Could you check a few things on this model? Use its own coordinates, in mm. Face numbers are marked on the shaded views. A direction names the side the tool comes from. Coordinates: 2 decimals unless noted, no trailing zeros. Write each loop counter-clockwise with the first axis right and the second up, starting at its lowest first coordinate (ties: lowest second). Pieces come first, ordered by that corner, then holes. Notation, with made-up numbers: (-28.75, -4) - (10.25, -4) arc R33 ccw to (10.25, 24) - close; hole circle Ø7 at (-23.5, 62). An arc over 180 degrees is marked (long way). Answer as a JSON object with one key per item and string values. Group by question number.
1) If we section it at D-D (z = -4.75): Write out the boundary of the cut face in (x, y) (3 decimals).
2) Will these pins go through, and if not, where does the flat tip stop? pin 1 Ø4 at (x, z) = (5, -6.5) entering from +Y (3 decimals); pin 2 Ø1 at (x, y) = (15.5, 6.5) entering from +Z (3 decimals).
3) If we section it at C-C (y = 1.75): State how many separate pieces and enclosed holes the cut face has, plus the area to 3 significant figures.
4) We'd pull the mould along X, two halves only. Please class the marked faces 3, 4 and 5: released by +X, released by -X, zero draft, split by the parting line, or undercut.
5) If we section it at A-A (x = 12.7): Write out the boundary of the cut face in (y, z) (1 decimal), plus the area to 3 significant figures.
6) Please list where these lines run through material, in increasing order: line 1 along X through (y, z) = (1, -4.5); line 2 along Y through (x, z) = (12.7, -11.65) (1 decimal); line 3 along Z through (x, y) = (19.05, 0.8) (3 decimals).
7) If we section it at B-B (y = 5.08): Write out the boundary of the cut face in (x, z) (1 decimal).
8) On a 3-axis mill with a long thin cutter (end or side, diameter ignored), from which of +Z, -Z, +X, -X, +Y, -Y can I reach the whole of each face in a straight line? I mean the marked faces 1 and 2. Say none if no direction works.
```python
from build123d import *

# Parameters (mm, degrees)
SKETCH1_W           = 25.4
SKETCH1_H           = 12.7
BOSS_EXTRUDE1_DEPTH = 3.175
SKETCH2_W           = 25.4
SKETCH2_H           = 3.175
BOSS_EXTRUDE2_DEPTH = 6.35
SKETCH3_R           = 0.9525
CUT_EXTRUDE1_DEPTH  = 30.952890094
SKETCH4_R           = 1.5875
CUT_EXTRUDE2_DEPTH  = 30.099355663


with BuildPart() as part:
    # Sketch1 → Boss-Extrude1 (new body)
    with BuildSketch(Plane(origin=(0, 0, 0), x_dir=(1, 0, 0), z_dir=(0, 1, 0))):
        with Locations((12.7, 6.35)):
            Rectangle(SKETCH1_W, SKETCH1_H)
    extrude(amount=BOSS_EXTRUDE1_DEPTH)

    # Sketch2 → Boss-Extrude2 (add)
    with BuildSketch(Plane(origin=(0, 3.175, 0), x_dir=(1, 0, 0), z_dir=(0, 1, 0))):
        with Locations((12.7, 11.1125)):
            Rectangle(SKETCH2_W, SKETCH2_H)
    extrude(amount=BOSS_EXTRUDE2_DEPTH)

    # Sketch3 → Cut-Extrude1 (cut, through all)
    with BuildSketch(Plane(origin=(0, 0, -12.7), x_dir=(-1, 0, 0), z_dir=(0, 0, -1))):
        with Locations((-12.7, 5.08)):
            Circle(SKETCH3_R)
    extrude(amount=-CUT_EXTRUDE1_DEPTH, mode=Mode.SUBTRACT)

    # Sketch4 → Cut-Extrude2 (cut, through all)
    with BuildSketch(Plane(origin=(0, 3.175, 0), x_dir=(1, 0, 0), z_dir=(0, 1, 0))):
        with Locations(Location((6.35, 4.7625, 0), (0, 0, 270))):
            Circle(SKETCH4_R)
        with Locations(Location((19.05, 4.7625, 0), (0, 0, 90))):
            Circle(SKETCH4_R)
    extrude(amount=-CUT_EXTRUDE2_DEPTH, mode=Mode.SUBTRACT)


solid = part.part
```
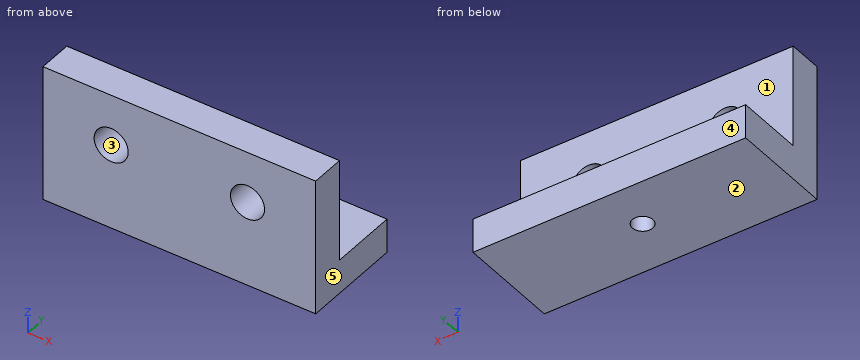
Here are the results:
{
 "1": {"outline": "(0, 0) - (4.763, 0) - (4.763, 3.175) - (0, 3.175) - close; (7.937, 0) - (17.463, 0) - (17.463, 3.175) - (7.937, 3.175) - close; (20.637, 0) - (25.4, 0) - (25.4, 3.175) - (20.637, 3.175) - close"},
 "2": {"pin 1": "stops at y = 3.175", "pin 2": "stops at z = -9.525"},
 "3": {"separate pieces": "1", "enclosed holes": "2", "area": "307 mm²"},
 "4": {"face 3": "undercut", "face 4": "zero draft", "face 5": "released by +X"},
 "5": {"outline": "(0, -12.7) - (4.1, -12.7) - (4.1, -9.5) - (3.2, -9.5) - (3.2, 0) - (0, 0) - close; (6, -12.7) - (9.5, -12.7) - (9.5, -9.5) - (6, -9.5) - close", "area": "54.4 mm²"},
 "6": {"line 1": "x = 0 to 4.78, 7.92 to 17.48, 20.62 to 25.4", "line 2": "y = 0 to 4.1, 6 to 9.5", "line 3": "z = -12.7 to -6.35, -3.175 to 0"},
 "7": {"outline": "(0, -12.7) - (11.7, -12.7) - (11.7, -9.5) - (0, -9.5) - close; (13.7, -12.7) - (25.4, -12.7) - (25.4, -9.5) - (13.7, -9.5) - close"},
 "8": {"face 1": "+Z, +X, -X, +Y", "face 2": "-Z, +X, -X, +Y, -Y"}
}
